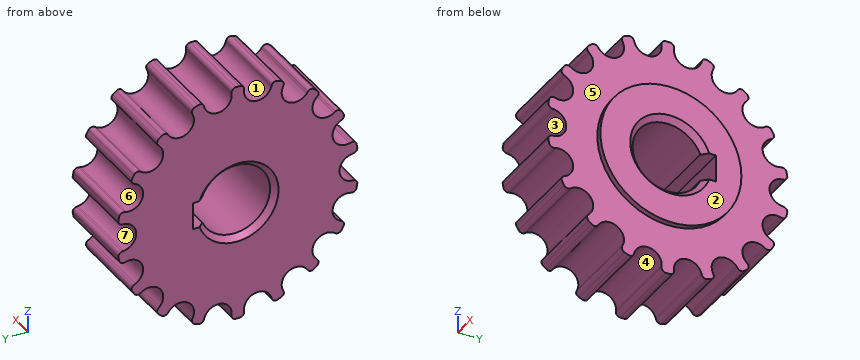
```python
from build123d import *

# Parameters (mm, degrees)
CHAMFER_1_SIZE           = 1
SKETCH_4_W               = 5
SKETCH_4_H               = 2.299999952
CUT_EXTRUDE_1_DEPTH      = 17
CUT_EXTRUDE_2_DEPTH      = 15
PATTERN_CIRCULAR_3_COUNT = 18


with BuildPart() as part:
    # Sketch 1 → Revolve 1 (revolve)
    with BuildSketch(Plane.XY):
        Polygon((0, 6.4838), (0, 22.234), (15, 22.234), (15, 12.9676), (16, 12.9676), (16, 6.4838), align=None)
    revolve(axis=Axis((0, 0, 0), (1, 0, 0)))

    # Chamfer 1
    chamfer_1_edges = [part.edges().sort_by_distance(p)[0] for p in [
        (0, -6.4838, 0),
        (16, -6.4838, 0),
    ]]
    chamfer(chamfer_1_edges, length=CHAMFER_1_SIZE)

    # Sketch 4 → Cut-Extrude 1 (cut, through all)
    with BuildSketch(Plane.ZY):
        with Locations((0, 7.132446168)):
            Rectangle(SKETCH_4_W, SKETCH_4_H)
    extrude(amount=-CUT_EXTRUDE_1_DEPTH, mode=Mode.SUBTRACT)

    # Sketch 6 → Cut-Extrude 2 (cut)
    with BuildSketch(Plane(origin=(0, 0, 0), x_dir=(0, 0, -1), z_dir=(1, 0, 0))):
        with BuildLine():
            Line((2.591680038, 21.283381802), (2.55084361, 20.950795787))
            ThreePointArc((2.55084361, 20.950795787), (0, 18.694), (-2.55084361, 20.950795787))
            Line((-2.55084361, 20.950795787), (-2.591680038, 21.283381802))
            ThreePointArc((-2.591680038, 21.283381802), (-2.896593224, 21.811367074), (-3.488238344, 21.95866456))
            ThreePointArc((-3.488238344, 21.95866456), (-3.872872102, 21.894100066), (-4.256314176, 21.822798758))
            Line((-4.256314176, 21.822798758), (-4.452962165, 23.4243681))
            ThreePointArc((-4.452962165, 23.4243681), (0, 23.843864891), (4.452962165, 23.4243681))
            Line((4.452962165, 23.4243681), (4.256314176, 21.822798758))
            ThreePointArc((4.256314176, 21.822798758), (3.872872102, 21.894100066), (3.488238344, 21.95866456))
            ThreePointArc((3.488238344, 21.95866456), (2.896593224, 21.811367074), (2.591680038, 21.283381802))
        make_face()
    cut_extrude_2 = extrude(amount=CUT_EXTRUDE_2_DEPTH, mode=Mode.SUBTRACT)

    # Pattern Circular 3: Cut-Extrude 2 ×18 about axis
    pattern_circular_3_axis = Axis((0, 0, 0), (1, 0, 0))
    for i in range(1, PATTERN_CIRCULAR_3_COUNT):
        add(cut_extrude_2.rotate(pattern_circular_3_axis, i * 360 / PATTERN_CIRCULAR_3_COUNT), mode=Mode.SUBTRACT)


solid = part.part
```
Here's how the part is built. I have some questions about the finished solid (model axes, mm). Face numbers are marked on the shaded views. A direction names the side the tool comes from. Round coordinates to 2 decimals unless told otherwise and drop trailing zeros. Order: outer loops, then holes, each group sorted by start corner. A loop starts at its lowest first (then second) coordinate and runs counter-clockwise, first axis right, second up. Notation, with made-up numbers: (-25.5, 24) -> (-20.5, 24) arc R10 cw to (-20.5, 29) -> close; hole circle Ø4 at (36, -39). An arc over 180 degrees is marked (long way). Use a Markdown table: item, result. Add a question column.
(1) Suppose I cut it at A-A, the plane z = 0. Please give me the cut outline in (x, y).
(2) I need wall thicknesses on line 1 along Z through (x, y) = (9.25, 0); line 2 along Y through (x, z) = (11, -16.5); line 3 along X through (y, z) = (1.5, -19.5). Which ranges of each line are inside material? Lowest first, please.
(3) For the marked faces 5, 6 and 7, which set-ups out of +Z, -Z, +X, -X, +Y, -Y let a thin tool reach every point of the face, with its end or its side?
(4) If we mould it in two halves opening along Y, with no side actions, what happens to the marked faces 1, 2, 3 and 4? For each: released by +Y, released by -Y, zero draft, split by the parting line, or undercut.
(5) Suppose I cut it at B-B, the plane y = 11.5. Please give me the cut outline in (x, z), and give its area (3 significant figures).
(6) For pin 1 Ø1 at (x, y) = (2.5, -14) entering from +Z; pin 2 Ø1.1 at (x, y) = (8.5, 7.5) entering from -Z; pin 3 Ø12 at (y, z) = (12.5, 16.5) entering from -X; pin 4 Ø1.5 at (x, z) = (4.5, 0.5) entering from -Y, each with a flat end and sliding along its axis, tell me the tip position at first contact or that it passes through.
Verdict:
| question | item | result |
|---|---|---|
| 1 | outline | (0, -18.69) -> (15, -18.69) -> (15, -12.97) -> (16, -12.97) -> (16, -7.48) -> (15, -6.48) -> (1, -6.48) -> (0, -7.48) -> close; (0, 8.28) -> (16, 8.28) -> (16, 12.97) -> (15, 12.97) -> (15, 18.69) -> (0, 18.69) -> close |
| 2 | line 1 | -22.23 to -6.48, 6.48 to 22.23 |
| 2 | line 2 | -14.79 to -12.35, -8.92 to 8.92, 12.35 to 14.79 |
| 2 | line 3 | 0 to 15 |
| 3 | face 5 | +X |
| 3 | face 6 | +X, -X |
| 3 | face 7 | +X, -X, +Y |
| 4 | face 1 | undercut |
| 4 | face 2 | zero draft |
| 4 | face 3 | released by -Y |
| 4 | face 4 | undercut |
| 5 | outline | (0, -16) -> (15, -16) -> (15, -5.99) -> (16, -5.99) -> (16, 5.99) -> (15, 5.99) -> (15, 16) -> (0, 16) -> close |
| 5 | area | 492 mm2 |
| 6 | pin 1 | z = 17.45 |
| 6 | pin 2 | z = -21.06 |
| 6 | pin 3 | x = 0 |
| 6 | pin 4 | y = -19.02 |
